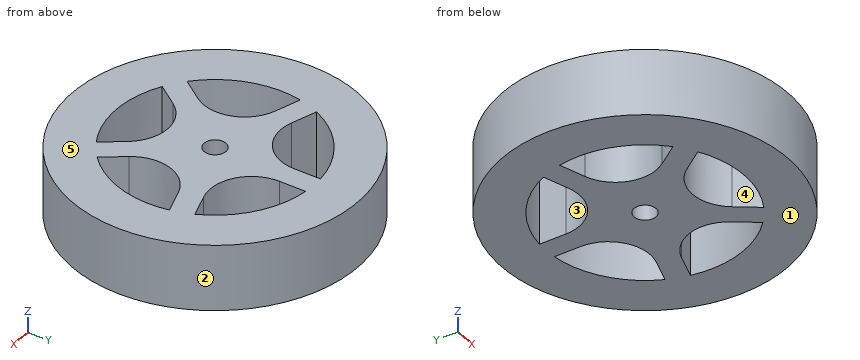
```python
from build123d import *

# Parameters (mm, degrees)
SKETCH_1_R      = 32.5
SKETCH_1_R_2    = 2.5
EXTRUDE_1_DEPTH = 15


with BuildPart() as part:
    # 草圖1 → 填料-伸長1 (new body)
    with BuildSketch(Plane.XY):
        Circle(SKETCH_1_R)
        Circle(SKETCH_1_R_2, mode=Mode.SUBTRACT)
        with BuildLine():
            Line((-2.5, 22.360679775), (-2.5, 16.360679775))
            ThreePointArc((-2.5, 16.360679775), (-6.369348392, 8.766655972), (-14.787388625, 7.433369381))
            Line((-14.787388625, 7.433369381), (-20.493727723, 9.287471347))
            ThreePointArc((-20.493727723, 9.287471347), (-13.225168177, 18.202882373), (-2.5, 22.360679775))
        make_face(mode=Mode.SUBTRACT)
        with BuildLine():
            Line((2.5, 22.360679775), (2.5, 16.360679775))
            ThreePointArc((2.5, 16.360679775), (6.369348392, 8.766655972), (14.787388625, 7.433369381))
            Line((14.787388625, 7.433369381), (20.493727723, 9.287471347))
            ThreePointArc((20.493727723, 9.287471347), (13.225168177, 18.202882373), (2.5, 22.360679775))
        make_face(mode=Mode.SUBTRACT)
        with BuildLine():
            Line((22.038812695, 4.532188766), (16.332473597, 2.678086799))
            ThreePointArc((16.332473597, 2.678086799), (10.305822184, -3.348564614), (11.639108775, -11.766604847))
            Line((11.639108775, -11.766604847), (15.165820289, -16.620706813))
            ThreePointArc((15.165820289, -16.620706813), (21.398771617, -6.952882373), (22.038812695, 4.532188766))
        make_face(mode=Mode.SUBTRACT)
        with BuildLine():
            Line((11.120735317, -19.559633074), (7.594023803, -14.705531108))
            ThreePointArc((7.594023803, -14.705531108), (0, -10.836182716), (-7.594023803, -14.705531108))
            Line((-7.594023803, -14.705531108), (-11.120735317, -19.559633074))
            ThreePointArc((-11.120735317, -19.559633074), (0, -22.5), (11.120735317, -19.559633074))
        make_face(mode=Mode.SUBTRACT)
        with BuildLine():
            Line((-15.165820289, -16.620706813), (-11.639108775, -11.766604847))
            ThreePointArc((-11.639108775, -11.766604847), (-10.305822184, -3.348564614), (-16.332473597, 2.678086799))
            Line((-16.332473597, 2.678086799), (-22.038812695, 4.532188766))
            ThreePointArc((-22.038812695, 4.532188766), (-21.398771617, -6.952882373), (-15.165820289, -16.620706813))
        make_face(mode=Mode.SUBTRACT)
    extrude(amount=EXTRUDE_1_DEPTH)


solid = part.part
```
For this review, take the finished solid that the model builds, in its own axes (mm). Face numbers are marked on the shaded views. A direction names the side the tool comes from. Give positions to 0.01 mm unless a question says otherwise; leave off trailing zeros. Write each loop counter-clockwise with the first axis right and the second up, starting at its lowest first coordinate (ties: lowest second). Pieces come first, ordered by that corner, then holes. Notation, with made-up numbers: M 18.25,5.5 L 60.25,5.5 A13 ccw 60.25,27.5 Z; hole C 32.25,54.25 d10. An arc over 180 degrees is marked long. Answer as a JSON object with one key per item and string values. Group by question number.
Item 1: Consider section A-A on x = 0. Write out the cut boundary in (y, z), plus the area to 3 significant figures.
Item 2: For probe 1 along Y at (x, z) = (0, 5.5); probe 2 along X at (y, z) = (14.5, 7.75); probe 3 along X at (y, z) = (11.5, 5.25), list the stretches that pass through material, from the lowest coordinate up. Write a range as [from, to].
Item 3: For pin 1 Ø3 at (y, z) = (20.5, 10) entering from -X; pin 2 Ø5 at (y, z) = (21, 7.5) entering from +X; pin 3 Ø6 at (y, z) = (-8.5, 8) entering from +X, all flat-tipped, find the tip position at first contact; note any pin that passes through.
Item 4: Consider section C-C on z = 8.5. Write out the cut boundary in (x, y).
Item 5: Consider section B-B on y = 21.5. Write out the cut boundary in (x, z).
Item 6: Consider section D-D on y = 0. Write out the cut boundary in (x, z).
Item 7: Draft analysis for pull direction Y (two halves, no side actions). For the marked faces 1, 2 and 3, state which applies: +Y half, -Y half, draft (parallel to the pull), parting line (faces both ways), or undercut.
Item 8: Tool access review of the marked faces 4 and 5: name each direction out of +Z, -Z, +X, -X, +Y, -Y from which nothing blocks a thin tool from reaching the whole face with its end or side.
Check result:
{
 "1": {"outline": "M -32.5,0 L -22.5,0 L -22.5,15 L -32.5,15 Z; M -10.84,0 L -2.5,0 L -2.5,15 L -10.84,15 Z; M 2.5,0 L 32.5,0 L 32.5,15 L 2.5,15 Z", "area": "725 mm^2"},
 "2": {"probe 1": "y = [-32.5, -22.5], [-10.84, -2.5], [2.5, 32.5]", "probe 2": "x = [-29.09, -17.2], [-2.69, 2.69], [17.2, 29.09]", "probe 3": "x = [-30.4, -19.34], [-3.86, 3.86], [19.34, 30.4]"},
 "3": {"pin 1": "stops at x = -26.37", "pin 2": "stops at x = 26.72", "pin 3": "stops at x = 32.03"},
 "4": {"outline": "C 0,0 d65; hole M -22.04,4.53 A22.5 ccw -15.17,-16.62 L -11.64,-11.77 A9.39 ccw -16.33,2.68 Z; hole M -20.49,9.29 L -14.79,7.43 A9.39 ccw -2.5,16.36 L -2.5,22.36 A22.5 ccw Z; hole M -11.12,-19.56 A22.5 ccw 11.12,-19.56 L 7.59,-14.71 A9.39 ccw -7.59,-14.71 Z; hole C 0,0 d5; hole M 2.5,16.36 A9.39 ccw 14.79,7.43 L 20.49,9.29 A22.5 ccw 2.5,22.36 Z; hole M 11.64,-11.77 L 15.17,-16.62 A22.5 ccw 22.04,4.53 L 16.33,2.68 A9.39 ccw Z"},
 "5": {"outline": "M -24.37,0 L -6.63,0 L -6.63,15 L -24.37,15 Z; M -2.5,0 L 2.5,0 L 2.5,15 L -2.5,15 Z; M 6.63,0 L 24.37,0 L 24.37,15 L 6.63,15 Z"},
 "6": {"outline": "M -32.5,0 L -22.5,0 L -22.5,15 L -32.5,15 Z; M -12.23,0 L -2.5,0 L -2.5,15 L -12.23,15 Z; M 2.5,0 L 12.23,0 L 12.23,15 L 2.5,15 Z; M 22.5,0 L 32.5,0 L 32.5,15 L 22.5,15 Z"},
 "7": {"face 1": "draft", "face 2": "parting line", "face 3": "undercut"},
 "8": {"face 4": "+Z, -Z", "face 5": "+Z, +X, -X, +Y, -Y"}
}
